from build123d import *

# Parameters (mm, degrees)
F1_R     = 1.5
F1_W     = 15
F1_H     = 13
F2_DEPTH = 3.4
F3_W     = 8
F3_H     = 0.95
F4_DEPTH = 18
F5_DEPTH = 18
F6_R     = 3
F7_R     = 3
F8_R     = 5
F9_R     = 5


with BuildPart() as f2:
    # F1 (on Front) → F2 (new body)
    with BuildSketch(Plane.XZ):
        Polygon((12.5, -22.5), (12.5, 22.5), (7.5, 22.5), (7.5, 9.5), (-7.5, 9.5), (-7.5, 22.5), (-12.5, 22.5), (-12.5, -22.5), align=None)
        with BuildLine():
            Line((7.5, 22.5), (12.5, 22.5))
            Line((12.5, 22.5), (7.5, 35.5))
            Line((7.5, 35.5), (7.5, 30.6180339887))
            ThreePointArc((7.5, 30.6180339887), (7.8693063938, 30.1123724357), (8, 29.5))
            ThreePointArc((8, 29.5), (7.8693063938, 28.8876275643), (7.5, 28.3819660113))
            Line((7.5, 28.3819660113), (7.5, 22.5))
        make_face()
        with BuildLine():
            Line((-7.5, 22.5), (7.5, 22.5))
            Line((7.5, 22.5), (7.5, 28.3819660113))
            ThreePointArc((7.5, 28.3819660113), (5, 29.5), (7.5, 30.6180339887))
            Line((7.5, 30.6180339887), (7.5, 35.5))
            Line((7.5, 35.5), (-7.5, 35.5))
            Line((-7.5, 35.5), (-7.5, 22.5))
        make_face()
        with Locations((0, 31)):
            Circle(F1_R, mode=Mode.SUBTRACT)
        Polygon((-12.5, 22.5), (-7.5, 22.5), (-7.5, 35.5), align=None)
        with Locations((0, 16)):
            Rectangle(F1_W, F1_H)
    extrude(amount=F2_DEPTH)

    # F3 (on face) → F4 (cut)
    with BuildSketch(Plane.XY.offset(35.5)):
        with Locations((0, -0.475)):
            Rectangle(F3_W, F3_H)
    extrude(amount=-F4_DEPTH, mode=Mode.SUBTRACT)

    # F3 (on face) → F5 (cut)
    with BuildSketch(Plane.XY.offset(35.5)):
        with Locations((0, -2.925)):
            Rectangle(F3_W, F3_H)
    extrude(amount=-F5_DEPTH, mode=Mode.SUBTRACT)

    # F6
    f6_edges = [f2.edges().sort_by_distance(p)[0] for p in [
        (-7.5, -1.7, 35.5),
    ]]
    fillet(f6_edges, radius=F6_R)

    # F7
    f7_edges = [f2.edges().sort_by_distance(p)[0] for p in [
        (7.5, -1.7, 35.5),
    ]]
    fillet(f7_edges, radius=F7_R)

    # F8
    f8_edges = [f2.edges().sort_by_distance(p)[0] for p in [
        (12.5, -1.7, 22.5),
    ]]
    fillet(f8_edges, radius=F8_R)

    # F9
    f9_edges = [f2.edges().sort_by_distance(p)[0] for p in [
        (-12.5, -1.7, 22.5),
    ]]
    fillet(f9_edges, radius=F9_R)


solid = f2.part
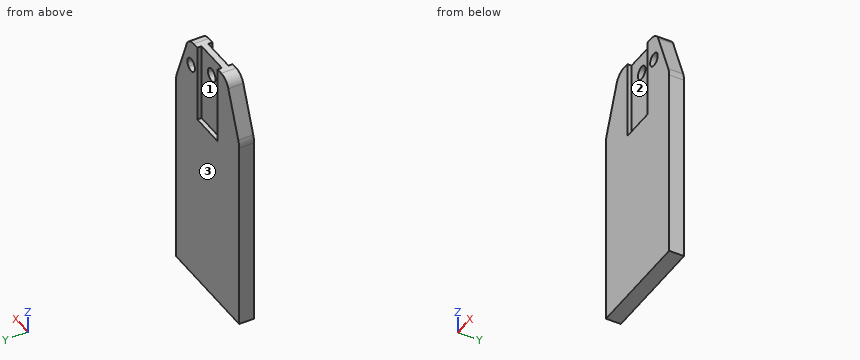
Input: part model. Units: mm. Frame: model coordinates. Face numbers are marked on the shaded views. A direction names the side the tool comes from. Coordinates: 2 decimals unless noted, no trailing zeros. Order: outer loops, then holes, each group sorted by start corner. A loop starts at its lowest first (then second) coordinate and runs counter-clockwise, first axis right, second up. Notation, with made-up numbers: M 24,9.25 L 52,9.25 A27 cw 52,45.25 Z; hole C 70.5,27.25 d8. An arc over 180 degrees is marked long. Answer in a Markdown table with one row per item.
(1) Section query B-B, the plane y = -1.5. Output: boundary loops of the cut face in (x, z).
Numbers:
| item | result |
|---|---|
| outline | M -12.5,-22.5 L 12.5,-22.5 L 12.5,21.57 A5 ccw 12.17,23.37 L 8.24,33.58 A3 ccw 5.44,35.5 L -5.44,35.5 A3 ccw -8.24,33.58 L -12.17,23.37 A5 ccw -12.5,21.57 Z; hole C 0,31 d3; hole C 6.5,29.5 d3 |
(2) Access query for the marked faces 1, 2 and 3. Directions: +Z, -Z, +X, -X, +Y, -Y. A direction counts if a zero-diameter tool reaches every point of the face in a straight line with its end or side. Return the directions, or none.
Numbers:
| item | result |
|---|---|
| face 1 | +Z, +Y |
| face 2 | +Z, -Y |
| face 3 | +Z, -Z, +X, -X, +Y |
(3) Material intervals for line 1 (Z direction, x = 5.5, y = -2); line 2 (Z direction, x = 3, y = -2.9); line 3 (Z direction, x = 0, y = -1.5), sorted ascending. Write a range as [from, to].
Numbers:
| item | result |
|---|---|
| line 1 | z = [-22.5, 28.38], [30.62, 35.5] |
| line 2 | z = [-22.5, 17.5] |
| line 3 | z = [-22.5, 29.5], [32.5, 35.5] |
(4) Contact query for flat-ended pins moving along their axis: pin 1 Ø3.5 at (x, z) = (0, 31) entering from +Y; pin 2 Ø1 at (x, y) = (1.5, -3) entering from +Z; pin 3 Ø2 at (y, z) = (-2, 27) entering from +X. Output: stop coordinate, or through.
Numbers:
| item | result |
|---|---|
| pin 1 | stops at y = -0.95 |
| pin 2 | stops at z = 17.5 |
| pin 3 | stops at x = 11.15 |
(5) Section query A-A, the plane x = 0. Output: boundary loops of the cut face in (y, z).
Numbers:
| item | result |
|---|---|
| outline | M -3.4,-22.5 L 0,-22.5 L 0,17.5 L -0.95,17.5 L -0.95,29.5 L -2.45,29.5 L -2.45,17.5 L -3.4,17.5 Z; M -2.45,32.5 L -0.95,32.5 L -0.95,35.5 L -2.45,35.5 Z |
(6) Section query C-C, the plane z = 18.5. Output: boundary loops of the cut face in (x, y), plus the area to 3 significant figures.
Numbers:
| item | result |
|---|---|
| outline | M -12.5,-3.4 L -4,-3.4 L -4,-2.45 L 4,-2.45 L 4,-3.4 L 12.5,-3.4 L 12.5,0 L 4,0 L 4,-0.95 L -4,-0.95 L -4,0 L -12.5,0 Z |
| area | 69.8 mm^2 |
(7) Section query D-D, the plane x = 6.5. Output: boundary loops of the cut face in (y, z).
Numbers:
| item | result |
|---|---|
| outline | M -3.4,-22.5 L 0,-22.5 L 0,28 L -3.4,28 Z; M -3.4,31 L 0,31 L 0,35.31 L -3.4,35.31 Z |
